from build123d import *

# Parameters (mm, degrees)
F0_R     = 25.4
F0_R_2   = 11
F1_DEPTH = 2


with BuildPart() as f1:
    # F0 (on Top) → F1 (new body, symmetric)
    with BuildSketch(Plane.XY):
        Circle(F0_R)
        with BuildLine():
            ThreePointArc((-9.090554, -18.173173), (-10.138809, -16.858575), (-9.813848, -15.208905))
            Line((-9.813848, -15.208905), (-8.129378, -12.890431))
            ThreePointArc((-8.129378, -12.890431), (-7.014806, -12.130407), (-5.671171, -12.251033))
            ThreePointArc((-5.671171, -12.251033), (-4.171729, -12.839263), (-2.612903, -13.244725))
            ThreePointArc((-2.612903, -13.244725), (-1.454977, -13.936905), (-1, -15.206906))
            Line((-1, -15.206906), (-1, -18.072698))
            ThreePointArc((-1, -18.072698), (-1.706753, -19.598316), (-3.327511, -20.0457))
            ThreePointArc((-3.327511, -20.0457), (-6.279225, -19.325468), (-9.090554, -18.173173))
        make_face(mode=Mode.SUBTRACT)
        with BuildLine():
            ThreePointArc((-18.036336, -9.359113), (-18.11169, -7.679431), (-16.87914, -6.535827))
            Line((-16.87914, -6.535827), (-14.15361, -5.650249))
            ThreePointArc((-14.15361, -5.650249), (-12.805172, -5.690506), (-11.78905, -6.577864))
            ThreePointArc((-11.78905, -6.577864), (-10.921729, -7.935101), (-9.898937, -9.179382))
            ThreePointArc((-9.898937, -9.179382), (-9.369008, -10.419979), (-9.747412, -11.71486))
            Line((-9.747412, -11.71486), (-11.431882, -14.033334))
            ThreePointArc((-11.431882, -14.033334), (-12.900393, -14.852167), (-14.474579, -14.26145))
            ThreePointArc((-14.474579, -14.26145), (-16.439225, -11.943796), (-18.036336, -9.359113))
        make_face(mode=Mode.SUBTRACT)
        with BuildLine():
            ThreePointArc((-20.092851, 3.029811), (-19.166522, 4.432995), (-17.497174, 4.633714))
            Line((-17.497174, 4.633714), (-14.771644, 3.748136))
            ThreePointArc((-14.771644, 3.748136), (-13.704397, 2.922975), (-13.403913, 1.607826))
            ThreePointArc((-13.403913, 1.607826), (-13.5, 0), (-13.403913, -1.607826))
            ThreePointArc((-13.403913, -1.607826), (-13.704397, -2.922975), (-14.771644, -3.748136))
            Line((-14.771644, -3.748136), (-17.497174, -4.633714))
            ThreePointArc((-17.497174, -4.633714), (-19.166522, -4.432995), (-20.092851, -3.029811))
            ThreePointArc((-20.092851, -3.029811), (-20.32, 0), (-20.092851, 3.029811))
        make_face(mode=Mode.SUBTRACT)
        Circle(F0_R_2, mode=Mode.SUBTRACT)
        with BuildLine():
            ThreePointArc((3.327511, -20.0457), (1.706753, -19.598316), (1, -18.072698))
            Line((1, -18.072698), (1, -15.206906))
            ThreePointArc((1, -15.206906), (1.454977, -13.936905), (2.612903, -13.244725))
            ThreePointArc((2.612903, -13.244725), (4.171729, -12.839263), (5.671171, -12.251033))
            ThreePointArc((5.671171, -12.251033), (7.014806, -12.130407), (8.129378, -12.890431))
            Line((8.129378, -12.890431), (9.813848, -15.208905))
            ThreePointArc((9.813848, -15.208905), (10.138809, -16.858575), (9.090554, -18.173173))
            ThreePointArc((9.090554, -18.173173), (6.279225, -19.325468), (3.327511, -20.0457))
        make_face(mode=Mode.SUBTRACT)
        with BuildLine():
            ThreePointArc((14.474579, -14.26145), (12.900393, -14.852167), (11.431882, -14.033334))
            Line((11.431882, -14.033334), (9.747412, -11.71486))
            ThreePointArc((9.747412, -11.71486), (9.369008, -10.419979), (9.898937, -9.179382))
            ThreePointArc((9.898937, -9.179382), (10.921729, -7.935101), (11.78905, -6.577864))
            ThreePointArc((11.78905, -6.577864), (12.805172, -5.690506), (14.15361, -5.650249))
            Line((14.15361, -5.650249), (16.87914, -6.535827))
            ThreePointArc((16.87914, -6.535827), (18.11169, -7.679431), (18.036336, -9.359113))
            ThreePointArc((18.036336, -9.359113), (16.439225, -11.943796), (14.474579, -14.26145))
        make_face(mode=Mode.SUBTRACT)
        with BuildLine():
            ThreePointArc((20.092851, -3.029811), (19.166522, -4.432995), (17.497174, -4.633714))
            Line((17.497174, -4.633714), (14.771644, -3.748136))
            ThreePointArc((14.771644, -3.748136), (13.704397, -2.922975), (13.403913, -1.607826))
            ThreePointArc((13.403913, -1.607826), (13.5, 0), (13.403913, 1.607826))
            ThreePointArc((13.403913, 1.607826), (13.704397, 2.922975), (14.771644, 3.748136))
            Line((14.771644, 3.748136), (17.497174, 4.633714))
            ThreePointArc((17.497174, 4.633714), (19.166522, 4.432995), (20.092851, 3.029811))
            ThreePointArc((20.092851, 3.029811), (20.32, 0), (20.092851, -3.029811))
        make_face(mode=Mode.SUBTRACT)
        with BuildLine():
            ThreePointArc((-14.474579, 14.26145), (-12.900393, 14.852167), (-11.431882, 14.033334))
            Line((-11.431882, 14.033334), (-9.747412, 11.71486))
            ThreePointArc((-9.747412, 11.71486), (-9.369008, 10.419979), (-9.898937, 9.179382))
            ThreePointArc((-9.898937, 9.179382), (-10.921729, 7.935101), (-11.78905, 6.577864))
            ThreePointArc((-11.78905, 6.577864), (-12.805172, 5.690506), (-14.15361, 5.650249))
            Line((-14.15361, 5.650249), (-16.87914, 6.535827))
            ThreePointArc((-16.87914, 6.535827), (-18.11169, 7.679431), (-18.036336, 9.359113))
            ThreePointArc((-18.036336, 9.359113), (-16.439225, 11.943796), (-14.474579, 14.26145))
        make_face(mode=Mode.SUBTRACT)
        with BuildLine():
            ThreePointArc((-9.090554, 18.173173), (-6.279225, 19.325468), (-3.327511, 20.0457))
            ThreePointArc((-3.327511, 20.0457), (-1.706753, 19.598316), (-1, 18.072698))
            Line((-1, 18.072698), (-1, 15.206906))
            ThreePointArc((-1, 15.206906), (-1.454977, 13.936905), (-2.612903, 13.244725))
            ThreePointArc((-2.612903, 13.244725), (-4.171729, 12.839263), (-5.671171, 12.251033))
            ThreePointArc((-5.671171, 12.251033), (-7.014806, 12.130407), (-8.129378, 12.890431))
            Line((-8.129378, 12.890431), (-9.813848, 15.208905))
            ThreePointArc((-9.813848, 15.208905), (-10.138809, 16.858575), (-9.090554, 18.173173))
        make_face(mode=Mode.SUBTRACT)
        with BuildLine():
            ThreePointArc((18.036336, 9.359113), (18.11169, 7.679431), (16.87914, 6.535827))
            Line((16.87914, 6.535827), (14.15361, 5.650249))
            ThreePointArc((14.15361, 5.650249), (12.805172, 5.690506), (11.78905, 6.577864))
            ThreePointArc((11.78905, 6.577864), (10.921729, 7.935101), (9.898937, 9.179382))
            ThreePointArc((9.898937, 9.179382), (9.369008, 10.419979), (9.747412, 11.71486))
            Line((9.747412, 11.71486), (11.431882, 14.033334))
            ThreePointArc((11.431882, 14.033334), (12.900393, 14.852167), (14.474579, 14.26145))
            ThreePointArc((14.474579, 14.26145), (16.439225, 11.943796), (18.036336, 9.359113))
        make_face(mode=Mode.SUBTRACT)
        with BuildLine():
            Line((1, 15.206906), (1, 18.072698))
            ThreePointArc((1, 18.072698), (1.706753, 19.598316), (3.327511, 20.0457))
            ThreePointArc((3.327511, 20.0457), (6.279225, 19.325468), (9.090554, 18.173173))
            ThreePointArc((9.090554, 18.173173), (10.138809, 16.858575), (9.813848, 15.208905))
            Line((9.813848, 15.208905), (8.129378, 12.890431))
            ThreePointArc((8.129378, 12.890431), (7.014806, 12.130407), (5.671171, 12.251033))
            ThreePointArc((5.671171, 12.251033), (4.171729, 12.839263), (2.612903, 13.244725))
            ThreePointArc((2.612903, 13.244725), (1.454977, 13.936905), (1, 15.206906))
        make_face(mode=Mode.SUBTRACT)
    extrude(amount=F1_DEPTH, both=True)

    # F2 (on Right) → F3 (revolve, cut)
    with BuildSketch(Plane.YZ):
        Polygon((-25.4442, 1.243426), (-25.4442, 0), (-23.4442, 0), align=None)
        Polygon((-23.4442, 0), (-25.4442, 0), (-25.4442, -1.243426), align=None)
    revolve(axis=Axis((0, 0, -6.003845), (0, 0, 1)), mode=Mode.SUBTRACT)


solid = f1.part
Design review of the part built by this model. Coordinates are the model's own, in mm. Give positions to 0.01 mm unless a question says otherwise; leave off trailing zeros. Write each loop counter-clockwise with the first axis right and the second up, starting at its lowest first coordinate (ties: lowest second). Pieces come first, ordered by that corner, then holes. Notation, with made-up numbers: M 65.5,-34 L 117.5,-34 A13 cw 117.5,-22 Z; hole C 76.5,-5 d5. An arc over 180 degrees is marked long. Return JSON: item names as keys, results as strings. Group by question number.
Item 1: Clearance check with flat-ended pins moving along their axes: pin 1 Ø1.5 at (x, z) = (17, -1.5) entering from +Y; pin 2 Ø2 at (x, z) = (-2.5, 1.5) entering from -Y; pin 3 Ø1.4 at (y, z) = (16.5, 0.5) entering from +X. State where each tip first meets the part, or that it passes through.
Item 2: Wall thickness on line 1 along X through (y, z) = (-12, 1.4); line 2 along X through (y, z) = (-15.5, 0.15); line 3 along X through (y, z) = (-8, 0.8): over which ranges is each line inside the solid? List them lowest first.
Item 3: Take a section at C-C (z = -0.6). Count the separate pieces of the cut face and the enclosed holes in it, plus the area to 3 significant figures.
Item 4: Take a section at B-B (x = 0). Give the boundary of the cut face in (y, z), plus the area to 3 significant figures.
Item 5: Take a section at A-A (y = 0). Give the boundary of the cut face in (x, z).
Item 6: The part is to be moulded in two halves that separate along Y. For faces 1 (the cylindrical face through (-6.32, 19.312, 0.028)), 2 (the flat face through (-16.115, -4.185, 0.028)), say which applies: pulls with the +Y half, pulls with the -Y half, needs draft (parallel to the pull), parting line crosses it, or undercut.
Return value:
{
 "1": {"pin 1": "stops at y = 19.52", "pin 2": "stops at y = -25.36", "pin 3": "stops at x = 19.39"},
 "2": {"line 1": "x = -22.39 to -16.4, -9.95 to 9.95, 16.4 to 22.39", "line 2": "x = -17.91 to -9.99, -1 to 1, 9.99 to 17.91", "line 3": "x = -23.4 to -18.21, -10.87 to -7.55, 7.55 to 10.87, 18.21 to 23.4"},
 "3": {"separate pieces": "1", "enclosed holes": "11", "area": "938 mm2"},
 "4": {"outline": "M -25.4,-2 L -11,-2 L -11,2 L -25.4,2 L -25.4,1.22 L -23.44,0 L -25.4,-1.22 Z; M 11,-2 L 25.4,-2 L 25.4,-1.22 L 23.44,0 L 25.4,1.22 L 25.4,2 L 11,2 Z", "area": "110 mm2"},
 "5": {"outline": "M -25.4,-2 L -20.32,-2 L -20.32,2 L -25.4,2 L -25.4,1.22 L -23.44,0 L -25.4,-1.22 Z; M -13.5,-2 L -11,-2 L -11,2 L -13.5,2 Z; M 11,-2 L 13.5,-2 L 13.5,2 L 11,2 Z; M 20.32,-2 L 25.4,-2 L 25.4,-1.22 L 23.44,0 L 25.4,1.22 L 25.4,2 L 20.32,2 Z"},
 "6": {"face 1": "undercut", "face 2": "undercut"}
}
